Geometry: final body of the model. Coordinates: model frame, mm. A direction names the side the tool comes from. Coordinates: 2 decimals unless noted, no trailing zeros. Write each loop counter-clockwise with the first axis right and the second up, starting at its lowest first coordinate (ties: lowest second). Pieces come first, ordered by that corner, then holes. Notation, with made-up numbers: (49, 78.25) -> (60, 78.25) arc R22 ccw to (60, 105.25) -> close; hole circle Ø10 at (-36.5, 22). An arc over 180 degrees is marked (long way). One line per item, written item: value.
```python
from build123d import *

# Parameters (mm, degrees)
PAD_DEPTH          = 12
FILLET_R           = 2
FILLET001_R        = 0.5
SKETCH001_R        = 4.375
PAD001_DEPTH       = 7
PAD002_DEPTH       = 12
CYLINDER_R         = 4.375
CYLINDER_DEPTH     = 56.568542
POLARPATTERN_COUNT = 4
SKETCH002_R        = 2.875
POCKET_DEPTH       = 7


with BuildPart() as part:
    # Sketch → Pad (new body)
    with BuildSketch(Plane.XY):
        with BuildLine():
            Line((-20, -16), (-20, 16))
            ThreePointArc((-16, 20), (-18.828427, 18.828427), (-20, 16))
            Line((-16, 20), (16, 20))
            ThreePointArc((20, 16), (18.828427, 18.828427), (16, 20))
            Line((20, 16), (20, -16))
            ThreePointArc((16, -20), (18.828427, -18.828427), (20, -16))
            Line((16, -20), (-16, -20))
            ThreePointArc((-20, -16), (-18.828427, -18.828427), (-16, -20))
        make_face()
    extrude(amount=PAD_DEPTH)

    # Fillet
    fillet_edges = [part.edges().sort_by_distance(p)[0] for p in [
        (20, 0, 12),
        (18.828427, -18.828427, 12),
        (0, -20, 12),
        (-18.828427, -18.828427, 12),
        (-20, 0, 12),
        (-18.828427, 18.828427, 12),
        (0, 20, 12),
        (18.828427, 18.828427, 12),
    ]]
    fillet(fillet_edges, radius=FILLET_R)

    # Fillet001
    fillet001_edges = [part.edges().sort_by_distance(p)[0] for p in [
        (0, 20, 0),
        (20, 0, 0),
        (18.828427, 18.828427, 0),
        (-18.828427, 18.828427, 0),
        (-20, 0, 0),
        (-18.828427, -18.828427, 0),
        (0, -20, 0),
        (18.828427, -18.828427, 0),
    ]]
    fillet(fillet001_edges, radius=FILLET001_R)

    # Sketch001 → Pad001 (join)
    with BuildSketch(Plane.XY):
        with Locations((-40, -40)):
            Circle(SKETCH001_R)
        with Locations((40, -40)):
            Circle(SKETCH001_R)
        with Locations((40, 40)):
            Circle(SKETCH001_R)
        with Locations((-40, 40)):
            Circle(SKETCH001_R)
    extrude(amount=-PAD001_DEPTH)

    # Sketch001 → Pad002 (join)
    with BuildSketch(Plane.XY):
        with Locations((-40, -40)):
            Circle(SKETCH001_R)
        with Locations((40, -40)):
            Circle(SKETCH001_R)
        with Locations((40, 40)):
            Circle(SKETCH001_R)
        with Locations((-40, 40)):
            Circle(SKETCH001_R)
    extrude(amount=PAD002_DEPTH)

    # Cylinder → Cylinder (join)
    with BuildSketch(Plane(origin=(0, 0, 7.625), x_dir=(0, 0, -1), z_dir=(0.707107, -0.707107, 0))):
        Circle(CYLINDER_R)
    cylinder = extrude(amount=CYLINDER_DEPTH)

    # PolarPattern: Cylinder ×4 about axis
    polarpattern_axis = Axis((0, 0, 0), (0, 0, 1))
    for i in range(1, POLARPATTERN_COUNT):
        add(cylinder.rotate(polarpattern_axis, i * 360 / POLARPATTERN_COUNT))

    # Sketch002 → Pocket (cut)
    with BuildSketch(Plane.XY):
        with Locations((-40, 40)):
            Circle(SKETCH002_R)
        with Locations((40, 40)):
            Circle(SKETCH002_R)
        with Locations((40, -40)):
            Circle(SKETCH002_R)
        with Locations((-40, -40)):
            Circle(SKETCH002_R)
    extrude(amount=-POCKET_DEPTH, mode=Mode.SUBTRACT)


solid = part.part
```
(1) Line query: line 1 (Y direction, x = -40, z = -3.5) (3 decimals); line 2 (Y direction, x = 34, z = 6); line 3 (X direction, y = 1.5, z = 6.75). Output: solid intervals per line, ascending. Write a range as [from, to].
Responses:
line 1: y = [-44.375, -42.875], [-37.125, -35.625], [35.625, 37.125], [42.875, 44.375]
line 2: y = [-39.74, -28.26], [28.26, 39.74]
line 3: x = [-20, 20]
(2) Reachability of faces 1 (the cylindrical face through (19.43, -0.22, 11.4)), 2 (the cylindrical face through (30.155, 26.39, 11.097)), 3 (the flat face through (-40, -40, 0)) from +Z, -Z, +X, -X, +Y, -Y: full face, straight path, thin tool, end or side. Return the list, or none.
Responses:
face 1: +Z, +X
face 2: none
face 3: -Z
(3) Section A-A (z = -5.5). Return the cut outline in (x, y) (3 decimals), then the cut area to 3 significant figures.
Responses:
outline: circle Ø8.75 at (-40, -40); circle Ø8.75 at (-40, 40); circle Ø8.75 at (40, -40); circle Ø8.75 at (40, 40); hole circle Ø5.75 at (-40, -40); hole circle Ø5.75 at (-40, 40); hole circle Ø5.75 at (40, -40); hole circle Ø5.75 at (40, 40)
area: 137 mm2
(4) First-contact query: pin 1 (8 mm diameter, centred on x = 2, z = 5.5, fed in from -Y); pin 2 (10 mm diameter, centred on y = -12.5, z = -2.5, fed in from +X); pin 3 (10 mm diameter, centred on y = 32.5, z = 1.5, fed in from +X). Flat tips, straight axial feed; report the tip coordinate or a pass-through.
Responses:
pin 1: stops at y = -20
pin 2: stops at x = 20
pin 3: stops at x = 43.59
(5) Pull-direction query (Y, two-part tool) for faces 4 (the cylindrical face through (-42.872, 40.126, -3.451)), 5 (the flat face through (-37, 39, -7)); classes: released by +Y, released by -Y, zero draft, split by the parting line, or undercut.
Responses:
face 4: undercut
face 5: zero draft
(6) Section B-B (x = -8). Return the cut outline in (y, z), then the cut area to 3 significant figures.
Responses:
outline: (-20, 0.5) arc R0.5 ccw to (-19.5, 0) -> (19.5, 0) arc R0.5 ccw to (20, 0.5) -> (20, 10) arc R2 ccw to (18, 12) -> (-18, 12) arc R2 ccw to (-20, 10) -> close
area: 478 mm2
